Verification items for the finished model (mm, model axes). A direction names the side the tool comes from. Give positions to 0.01 mm unless a question says otherwise; leave off trailing zeros. Order: outer loops, then holes, each group sorted by start corner. A loop starts at its lowest first (then second) coordinate and runs counter-clockwise, first axis right, second up. Notation, with made-up numbers: (-31, -21.75) - (-18, -21.75) arc R9 ccw to (-18, -9.75) - close; hole circle Ø5 at (14.5, 65). An arc over 180 degrees is marked (long way). Answer as a JSON object with one key per item and string values. Group by question number.
(1) Access from +Z, -Z, +X, -X, +Y, -Y to the whole of each face (thin tool, end or side, straight path). Record for faces 1 (the face through (-17.15, -15.07, 23.01)), 2 (the face through (10, 15, 40)), 3 (the face through (-20, 15, 20)), 4 (the face through (-10, -15, 15)), 5 (the face through (0, 10, 22)).
(2) Section check D-D (y = -14.5). Record the boundary of the cut face in (x, z), then the cut area to 3 significant figures.
(3) Depth check by flat-ended pin: pin 1 Ø5 at (x, y) = (-27.5, -16.5) entering from +Z; pin 2 Ø10 at (x, y) = (-7.5, -6) entering from +Z; pin 3 Ø8 at (x, z) = (19, 33) entering from -Y. Enter the tip coordinate at first touch or a pass-through.
(4) Thickness scan on line 1 (Z direction, x = 10, y = 13.25); line 2 (Y direction, x = -21.5, z = 22.5); line 3 (Z direction, x = -19, y = -9). Record the ranges inside material, lowest first.
(5) Mould release check, pull along Y, two halves, no side actions. Record for faces 6 (the face through (-7, -20, 8)), 7 (the face through (-22, -10, 18)), 8 (the face through (-30, 0, 8)), 9 (the face through (0, 20, 16)): +Y half, -Y half, draft (parallel to the pull), parting line (faces both ways), or undercut.
(6) Section check A-A (y = 11). Record the boundary of the cut face in (x, z), then the cut area to 3 significant figures.
(7) Section check B-B (x = 4.5). Record the boundary of the cut face in (y, z), then the cut area to 3 significant figures.
(8) Section check C-C (z = 27.5). Record the boundary of the cut face in (x, y), then the cut area to 3 significant figures.
```python
from build123d import *

# Parameters (mm, degrees)
F0_W      = 60
F0_H      = 40
F1_DEPTH  = 10
F2_W      = 60
F2_H      = 10
F3_DEPTH  = 10
F5_DEPTH  = 10
F7_DEPTH  = 10
F8_W      = 20
F8_H      = 10
F9_DEPTH  = 20
F11_DEPTH = 10


with BuildPart() as f1:
    # F0 (on Top) → F1 (new body)
    with BuildSketch(Plane.XY):
        Rectangle(F0_W, F0_H)
    extrude(amount=F1_DEPTH)

    # F2 (on face) → F3 (join)
    with BuildSketch(Plane.XY.offset(10)):
        with Locations((0, 15)):
            Rectangle(F2_W, F2_H)
    extrude(amount=F3_DEPTH)

    # F4 (on face) → F5 (join)
    with BuildSketch(Plane.XZ.offset(-10)):
        with BuildLine():
            Line((-10, 20), (30, 20))
            ThreePointArc((30, 20), (10, 40), (-10, 20))
        make_face()
    extrude(amount=-F5_DEPTH)

    # F6 (on face) → F7 (cut)
    with BuildSketch(Plane.XZ.offset(-10)):
        with BuildLine():
            ThreePointArc((10, 10), (17.071068, 12.928932), (20, 20))
            ThreePointArc((20, 20), (2.928932, 27.071068), (10, 10))
        make_face()
    extrude(amount=-F7_DEPTH, mode=Mode.SUBTRACT)

    # F8 (on face) → F9 (join)
    with BuildSketch(Plane.XY.offset(10)):
        with Locations((-20, -15)):
            Rectangle(F8_W, F8_H)
    extrude(amount=F9_DEPTH)

    # F10 (on face) → F11 (cut)
    with BuildSketch(Plane.XZ.offset(20)):
        with BuildLine():
            Line((-10, 30), (-20, 30))
            ThreePointArc((-20, 30), (-17.071068, 22.928932), (-10, 20))
            Line((-10, 20), (-10, 30))
        make_face()
    extrude(amount=-F11_DEPTH, mode=Mode.SUBTRACT)


solid = f1.part
```
Solutions:
{
 "1": {"face 1": "+Z, +X, +Y, -Y", "face 2": "+Z, +Y, -Y", "face 3": "+Z, -X, +Y", "face 4": "+Z, +X, -Y", "face 5": "+Z, +X, -X"},
 "2": {"outline": "(-30, 0) - (30, 0) - (30, 10) - (-10, 10) - (-10, 20) arc R10 cw to (-20, 30) - (-30, 30) - close", "area": "921 mm2"},
 "3": {"pin 1": "stops at z = 30", "pin 2": "stops at z = 20.01", "pin 3": "stops at y = 10"},
 "4": {"line 1": "z = 0 to 10, 30 to 40", "line 2": "y = -20 to -10", "line 3": "z = 0 to 10"},
 "5": {"face 6": "-Y half", "face 7": "undercut", "face 8": "draft", "face 9": "+Y half"},
 "6": {"outline": "(-30, 0) - (30, 0) - (30, 20) arc R20 ccw to (-10, 20) - (-30, 20) - close; hole circle Ø20 at (10, 20)", "area": "1,510 mm2"},
 "7": {"outline": "(-20, 0) - (20, 0) - (20, 11.65) - (10, 11.65) - (10, 10) - (-20, 10) - close; (10, 28.35) - (20, 28.35) - (20, 39.23) - (10, 39.23) - close", "area": "525 mm2"},
 "8": {"outline": "(-30, -20) - (-19.68, -20) - (-19.68, -10) - (-30, -10) - close; (-8.54, 10) - (3.39, 10) - (3.39, 20) - (-8.54, 20) - close; (16.61, 10) - (28.54, 10) - (28.54, 20) - (16.61, 20) - close", "area": "342 mm2"}
}
